Input: part model. Units: mm. Frame: model coordinates. Face numbers are marked on the shaded views. A direction names the side the tool comes from. Coordinates: 2 decimals unless noted, no trailing zeros. Loops run counter-clockwise (first coordinate to the right, second up) from the corner with the lowest first, then second, coordinate; pieces in that order, holes last.
```python
from build123d import *

# Parameters (mm, degrees)
F0_W     = 13.97
F0_H     = 99.06
F1_DEPTH = 76.2
F2_T     = -2.54
F3_R     = 8.994347
F4_DEPTH = 118.618


with BuildPart() as f1:
    # F0 (on Top) → F1 (new body)
    with BuildSketch(Plane.XY):
        Rectangle(F0_W, F0_H)
    extrude(amount=-F1_DEPTH)

    # F2
    f2_openings = [f1.faces().sort_by_distance(p)[0] for p in [
        (0, 0, -76.2),
        (0, 49.53, -38.1),
        (0, -49.53, -38.1),
    ]]
    offset(amount=F2_T, openings=f2_openings)

    # F3 (on face) → F4 (cut)
    with BuildSketch(Plane(origin=(-6.985, 0, 0), x_dir=(0, -1, 0), z_dir=(-1, 0, 0))):
        with Locations((0, -32.869287)):
            Circle(F3_R)
    extrude(amount=-F4_DEPTH, mode=Mode.SUBTRACT)


solid = f1.part
```
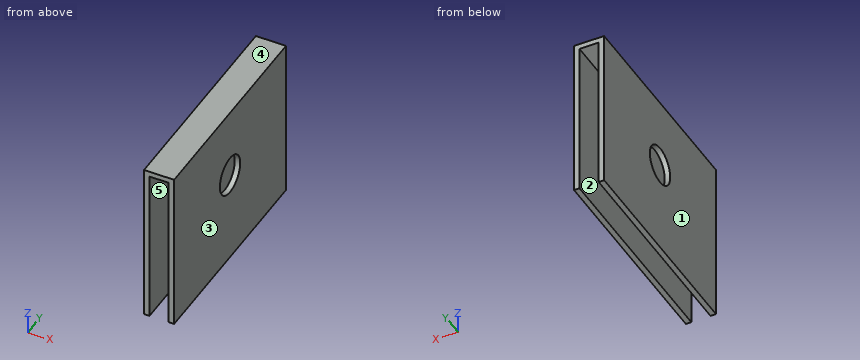
Item 1: Mould query, pull axis X, two halves, no side actions, for the marked faces 3, 4 and 5. Classes: +X half, -X half, draft (parallel to the pull), parting line (faces both ways), or undercut.
Result:
face 3: +X half
face 4: draft
face 5: undercut
Item 2: Section query B-B (z = -15). Output: boundary loops of the cut face in (x, y) (3 decimals).
Result:
outline: (-6.985, -49.53) - (-4.445, -49.53) - (-4.445, 49.53) - (-6.985, 49.53) - close; (4.445, -49.53) - (6.985, -49.53) - (6.985, 49.53) - (4.445, 49.53) - close
Item 3: Line query: L1, parallel to Z at x = -5.05, y = 0; L2, parallel to X at y = -32, z = -67 (3 decimals); L3, parallel to Z at x = 1.5, y = 15.5. Output: solid intervals per line, ascending.
Result:
L1: z = -76.2 to -41.86, -23.87 to 0
L2: x = -6.985 to -4.445, 4.445 to 6.985
L3: z = -2.54 to 0
Item 4: Section query A-A (y = 0). Output: boundary loops of the cut face in (x, z) (3 decimals), then the cut area to 3 significant figures.
Result:
outline: (-6.985, -76.2) - (-4.445, -76.2) - (-4.445, -41.864) - (-6.985, -41.864) - close; (-6.985, -23.875) - (-4.445, -23.875) - (-4.445, -2.54) - (4.445, -2.54) - (4.445, -23.875) - (6.985, -23.875) - (6.985, 0) - (-6.985, 0) - close; (4.445, -76.2) - (6.985, -76.2) - (6.985, -41.864) - (4.445, -41.864) - close
area: 318 mm2
Item 5: Reachability of the marked faces 1 and 2 from +Z, -Z, +X, -X, +Y, -Y: full face, straight path, thin tool, end or side. Return the list, or none.
Result:
face 1: +Z, -Z, -X, +Y, -Y
face 2: -Z, +Y, -Y
Item 6: Section query C-C (y = -19). Output: boundary loops of the cut face in (x, z) (3 decimals), then the cut area to 3 significant figures.
Result:
outline: (-6.985, -76.2) - (-4.445, -76.2) - (-4.445, -2.54) - (4.445, -2.54) - (4.445, -76.2) - (6.985, -76.2) - (6.985, 0) - (-6.985, 0) - close
area: 410 mm2
Item 7: Contact query for flat-ended pins moving along their axis: P1, Ø1.5, axis at x = -4, y = -14, coming from the -Z side; P2, Ø4, axis at x = 0.5, y = -5.5, coming from the -Z side; P3, Ø14.5, axis at y = 0, z = -32.87, coming from the -X side. Output: stop coordinate, or through.
Result:
P1: stops at z = -76.2
P2: stops at z = -2.54
P3: passes through
Item 8: Section query D-D (x = 5.75). Output: boundary loops of the cut face in (y, z), then the cut area to 3 significant figures.
Result:
outline: (-49.53, -76.2) - (49.53, -76.2) - (49.53, 0) - (-49.53, 0) - close; hole circle Ø17.99 at (0, -32.87)
area: 7,290 mm2
